```python
from build123d import *

# Parameters (mm, degrees)
SKETCH1_W                 = 25.4
SKETCH1_H                 = 12.7
BOSS_EXTRUDE1_DEPTH       = 62.738
F_2_56_TAPPED_HOLE1_D     = 1.778
F_2_56_TAPPED_HOLE1_DEPTH = 10.8204
F_2_56_TAPPED_HOLE1_TIP   = 0.53416509
F_8_32_TAPPED_HOLE1_D     = 3.4544
F_8_32_TAPPED_HOLE1_DEPTH = 10.70864
F_8_32_TAPPED_HOLE1_TIP   = 1.037806461


with BuildPart() as part:
    # Sketch1 → Boss-Extrude1 (new body)
    with BuildSketch(Plane(origin=(0, 0, 0), x_dir=(1, 0, 0), z_dir=(0, 1, 0))):
        with Locations((12.7, -6.35)):
            Rectangle(SKETCH1_W, SKETCH1_H)
    extrude(amount=BOSS_EXTRUDE1_DEPTH)

    # #2-56 Tapped Hole1
    with Locations(Plane(origin=(0, 0, 0), x_dir=(-1, 0, 0), z_dir=(0, -1, 0))):
        with Locations((-3.175, -6.35), (-22.225, -6.35)):
            Hole(F_2_56_TAPPED_HOLE1_D / 2, depth=F_2_56_TAPPED_HOLE1_DEPTH)
            with Locations((0, 0, -(F_2_56_TAPPED_HOLE1_DEPTH + F_2_56_TAPPED_HOLE1_TIP / 2))):  # 118° drill point
                Cone(0, F_2_56_TAPPED_HOLE1_D / 2, F_2_56_TAPPED_HOLE1_TIP, mode=Mode.SUBTRACT)

    # #8-32 Tapped Hole1
    with Locations(Plane(origin=(0, 62.738, 0), x_dir=(1, 0, 0), z_dir=(0, 1, 0))):
        with Locations((6.35, -6.35), (19.05, -6.35)):
            Hole(F_8_32_TAPPED_HOLE1_D / 2, depth=F_8_32_TAPPED_HOLE1_DEPTH)
            with Locations((0, 0, -(F_8_32_TAPPED_HOLE1_DEPTH + F_8_32_TAPPED_HOLE1_TIP / 2))):  # 118° drill point
                Cone(0, F_8_32_TAPPED_HOLE1_D / 2, F_8_32_TAPPED_HOLE1_TIP, mode=Mode.SUBTRACT)


solid = part.part
```
Model file for the job. Use its own axes, mm. A direction names the side the tool comes from. Round coordinates to 2 decimals unless told otherwise and drop trailing zeros. Put each result on its own line as item: value.
Item 1: Tool access for faces 1 (the flat face through (13, 31, 0)), 2 (the cylindrical face through (2.982, 5.486, 7.218)), 3 (the cylindrical face through (5.421, 57.309, 4.894)): list every direction of +Z, -Z, +X, -X, +Y, -Y with a clear straight run to the whole face (end or side of a thin tool).
Responses:
face 1: -Z, +X, -X, +Y, -Y
face 2: -Y
face 3: +Y
Item 2: Probe L1, parallel to X at y = 59.75, z = 6.35; L2, parallel to Y at x = 6.25, z = 7.5. List the from-to ranges inside material, lowest first. Write a range as from..to.
Responses:
L1: 0..4.62, 8.08..17.32, 20.78..25.4
L2: 0..51.69
Item 3: Flat gauge pins, fed straight in: P1, Ø3, axis at x = 19.05, z = 6.35, coming from the +Y side; P2, Ø5, axis at x = 10.5, z = 10.5, coming from the -Y side. Where does each tip first touch, or does it go through?
Responses:
P1: y = 51.89
P2: y = 0
Item 4: Mould opens along X. For faces 4 (the conical face through (3.028, 11.262, 6.304)), 5 (the flat face through (0, 31, 6)), 6 (the flat face through (13, 0, 6)) say: +X half, -X half, draft (parallel to the pull), parting line (faces both ways), or undercut.
Responses:
face 4: undercut
face 5: -X half
face 6: draft
